Autodesk Inventor part; units mm, degrees
ref_plane "YZ Plane" through (0, 0, 0) normal (1, 0, 0) x (0, 1, 0)
ref_plane "XZ Plane" through (0, 0, 0) normal (0, 1, 0) x (-1, 0, 0)
ref_plane "XY Plane" through (0, 0, 0) normal (0, 0, 1) x (1, 0, 0)
sketch "Sketch1" plane through (0, 0, 0) normal (0, 1, 0) x (-1, 0, 0)
  circle A0 centre (0, 0) radius 11 construction
  circle A1 centre (0, 0) radius 3.75
  circle A2 centre (0, 0) radius 7.875 construction
  line L0 (16.292, 0) -> (-19, 0) construction
  line L1 (0, 21) -> (0, -27.3544) construction
  line L2 (0, -21) -> (21, -21)
  line L3 (0, -21) -> (-21, -21)
  line L4 (0, 0) -> (21, -21) construction
  circle A3 centre (5.5685, -5.5685) radius 0.75
  circle A4 centre (-5.5685, -5.5685) radius 0.75
  circle A5 centre (5.5685, 5.5685) radius 0.75
  circle A6 centre (-5.5685, 5.5685) radius 0.75
  line L5 (-25, -21) -> (-21, -21)
  line L6 (25, -21) -> (21, -21)
  circle A7 centre (23, -14) radius 1
  circle A8 centre (-23, -14) radius 1
  line L7 (-25, 42) -> (25, 42)
  line L8 (25, -21) -> (25, 42)
  line L9 (21, -21) -> (21, 42)
  line L10 (-21, -21) -> (-21, 42)
  line L11 (-25, -21) -> (-25, 42)
  line L12 (25, 10.5) -> (-25, 10.5) construction
  circle A9 centre (23, 35) radius 1
  circle A10 centre (-23, 35) radius 1
  circle A11 centre (23, 10.5) radius 1
  circle A12 centre (-23, 10.5) radius 1
  circle A13 centre (5.5685, 5.5685) radius 1.5
  circle A14 centre (5.5685, -5.5685) radius 1.5
  circle A15 centre (-5.5685, 5.5685) radius 1.5
  circle A16 centre (-5.5685, -5.5685) radius 1.5
  dimension "d8" = 15.75
  dimension "d2" = 7.5
  dimension "d4" = 22
  dimension "d17" = 21
  dimension "d26" = 1.5
  dimension "d38" = 63
  dimension "d39" = 21
  dimension "d40" = 2
  dimension "d41" = 2
  dimension "d53" = 3
extrude "Extrusion9" add sketch "Sketch1" along normal blind 45 contours A1 | L3 L10 L7 L9 L2 | A3 | A4 | A5 | A6 | A13 | A14 | A15 | A16
extrude "Extrusion10" add sketch "Sketch1" along normal blind 27.5 contours L9 L7 L8 L6 | L5 L11 L7 L10
extrude "Extrusion11" cut sketch "Sketch1" along normal blind 17.5 contours L9 L7 L8 L6 | L5 L11 L7 L10
extrude "Extrusion13" cut sketch "Sketch1" along normal blind 6 contours A1 | A3 | A4 | A5 | A6 | A13 | A14 | A15 | A16
extrude "Extrusion15" add sketch "Sketch1" along normal blind 3.5 contours A13 | A14 | A15 | A16
sketch "Sketch5" plane through (-21, 45, 42) normal (0, 0, 1) x (1, 0, 0)
  line L0 (0, -45) -> (42, -45) construction
  line L1 (0, -17.5) -> (0, 0) construction
  line L2 (42, -45) -> (0, -45) construction
  line L3 (0, -45) -> (0, 0) construction
  line L4 (0, 0) -> (42, 0) construction
  line L5 (42, 0) -> (42, -45) construction
  line L6 (42, 0) -> (0, -45) construction
  line L7 (0, 0) -> (42, 0) construction
  line L8 (0, 0) -> (42, -45) construction
  circle A0 centre (21, -22.5) radius 18.5
  line L9 (-4, -27.5) -> (-4, -17.5) construction
  line L10 (-4, -22.5) -> (45.9746, -22.5) construction
  line L11 (-4, -23.5) -> (45.9746, -23.5) construction
  line L12 (45.9746, -23.5) -> (45.9746, -45) construction
  line L13 (45.9746, -45) -> (-4, -45) construction
  line L14 (-4, -45) -> (-4, -23.5) construction
  line L15 (-4, -21.5) -> (46, -21.5) construction
  line L16 (46, -21.5) -> (46, 0) construction
  line L17 (46, 0) -> (-4, 0) construction
  line L18 (-4, 0) -> (-4, -21.5) construction
  line L19 (-4, -21.5) -> (45.9746, -21.5) construction
  line L20 (45.9746, -21.5) -> (45.9746, -23.5) construction
  line L21 (45.9746, -23.5) -> (-4, -23.5) construction
  line L22 (-4, -23.5) -> (-4, -21.5) construction
  line L23 (10.2856, -7.4185) -> (31.7144, -7.4185)
  line L24 (5.9185, -11.7856) -> (5.9185, -33.2144)
  line L25 (36.0815, -11.7856) -> (36.0815, -33.2144)
  circle A1 centre (21, -22.5) radius 13.5 construction
  line L26 (21, -22.5) -> (38.8515, -22.5) construction
  line L27 (34.0815, -9.4185) -> (7.9185, -35.5815) construction
  line L28 (21, -45) -> (21, 0) construction
  line L29 (7.9185, -9.4185) -> (34.0815, -35.5815) construction
  line L30 (7.9185, -9.4185) -> (34.0815, -9.4185) construction
  line L31 (7.9185, -9.4185) -> (7.9185, -35.5815) construction
  line L32 (34.0815, -35.5815) -> (34.0815, -9.4185) construction
  circle A2 centre (4.5, -40.1786) radius 1
  circle A3 centre (37.5, -40.1786) radius 1
  circle A4 centre (4.5, -4.8214) radius 1
  circle A5 centre (37.5, -4.8214) radius 1
  dimension "d58" = 37
  dimension "d61" = 1
  dimension "d62" = 1
  dimension "d70" = 27
  dimension "d73" = 2
  dimension "d74" = 45
  dimension "d75" = 2
  dimension "d76" = 2
  dimension "d77" = 42
  dimension "d78" = 45
  dimension "d79" = 2
  dimension "d80" = 4.5
extrude "Extrusion16" cut sketch "Sketch5" against normal blind 62 contours L25 A0 L24 L23
extrude "Extrusion18" cut sketch "Sketch5" against normal blind 46 contours A0 L25 | L23 A0 | A0 L24
extrude "Extrusion19" cut sketch "Sketch5" against normal blind 5 contours A2 | A3 | A4 | A5
equation "\"d41\" = d40"
properties part number "engine_connector_sleeve"
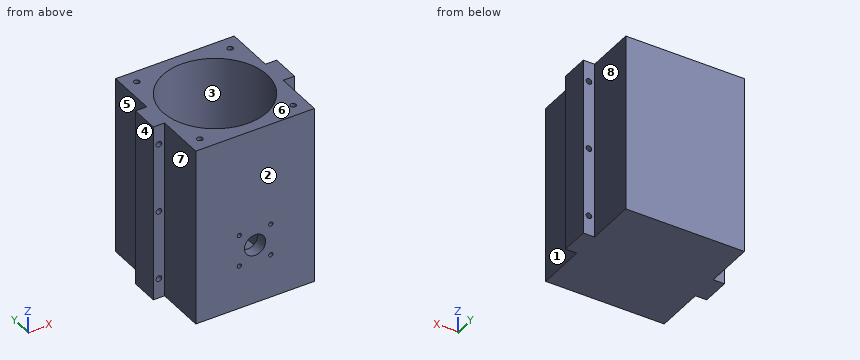
CAD build for the part. Positions are in the model's coordinates, mm. Face numbers are marked on the shaded views. A direction names the side the tool comes from. Give positions to 0.01 mm unless a question says otherwise; leave off trailing zeros. Order: outer loops, then holes, each group sorted by start corner. A loop starts at its lowest first (then second) coordinate and runs counter-clockwise, first axis right, second up. Notation, with made-up numbers: M 21,72 L 64,72 A24 cw 64,82 Z; hole C 2,50.25 d11. An arc over 180 degrees is marked long. Put each result on its own line as item: value. Start each with the question number.
(1) Saw through at C-C, the plane z = -14. Write the cut outline in (x, y), then the cut area to 3 significant figures.
(2) Which spindle directions (+Z, -Z, +X, -X, +Y, -Y) get a long thin tool onto all of the face, cutting with end or side? Do the marked faces 4, 5, 6, 7 and 8. Say none if no direction does.
(3) Mould opens along X. For the marked faces 1, 2 and 3 say: +X half, -X half, draft (parallel to the pull), parting line (faces both ways), or undercut.
(4) Drill centre lines: line 1 along Z through (x, y) = (-23, 21.5); line 2 along X through (y, z) = (24.5, -7); line 3 along Y through (x, z) = (-8, 33). Where is each one in solid material? Low to high.
(5) Saw through at B-B, the plane y = 22.5. Write the cut outline in (x, z).
(6) Saw through at A-A, the plane z = 10.5. Write the cut outline in (x, y), then the cut area to 3 significant figures.
(7) Saw through at D-D, the plane x = -9. Write the cut outline in (y, z).
(8) Flat gauge pins, fed straight in: pin 1 Ø5 at (y, z) = (39, 11.5) entering from +X; pin 2 Ø1 at (x, y) = (5, 34.5) entering from +Z; pin 3 Ø1.8 at (x, y) = (16.5, 4.82) entering from +Z. Where does each tip first touch, or does it go through?
Check result:
1. outline: M -25,17.5 L -24,17.5 L -24,27.5 L -25,27.5 Z; M -22,17.5 L -21,17.5 L -21,0 L 21,0 L 21,17.5 L 22,17.5 L 22,27.5 L 21,27.5 L 21,45 L -21,45 L -21,27.5 L -22,27.5 Z; M 24,17.5 L 25,17.5 L 25,27.5 L 24,27.5 Z; hole M -15.08,11.79 A18.5 ccw 15.08,11.79 L 15.08,33.21 A18.5 ccw 10.71,37.58 L -10.71,37.58 A18.5 ccw -15.08,33.21 Z
1. area: 1,000 mm2
2. face 4: +Z, -Z, -X, +Y, -Y
2. face 5: +Z, -Z, -X, +Y
2. face 6: +Z, +X, -X, +Y, -Y
2. face 7: +Z, -Z, -X, -Y
2. face 8: +Z, -Z, +X, +Y
3. face 1: +X half
3. face 2: draft
3. face 3: undercut
4. line 1: z = -21 to -15, -13 to 9.5, 11.5 to 34, 36 to 42
4. line 2: x = -25 to -15.08, 15.08 to 25
4. line 3: y = 0 to 5.82, 39.18 to 45
5. outline: M -25,-21 L 25,-21 L 25,42 L 18.5,42 L 18.5,-4 L 15.08,-4 L 15.08,-20 L -15.08,-20 L -15.08,-4 L -18.5,-4 L -18.5,42 L -25,42 Z; hole C -23,-14 d2; hole C -23,10.5 d2; hole C -23,35 d2; hole C 23,-14 d2; hole C 23,10.5 d2; hole C 23,35 d2
6. outline: M -25,17.5 L -24,17.5 L -24,27.5 L -25,27.5 Z; M -22,17.5 L -21,17.5 L -21,0 L 21,0 L 21,17.5 L 22,17.5 L 22,27.5 L 21,27.5 L 21,45 L -21,45 L -21,27.5 L -22,27.5 Z; M 24,17.5 L 25,17.5 L 25,27.5 L 24,27.5 Z; hole C 0,22.5 d37
6. area: 855 mm2
7. outline: M 0,-21 L 45,-21 L 45,42 L 38.66,42 L 38.66,-4 L 37.58,-4 L 37.58,-20 L 6.34,-20 L 6.34,42 L 0,42 Z
8. pin 1: stops at x = 21
8. pin 2: stops at z = -20
8. pin 3: stops at z = 37
